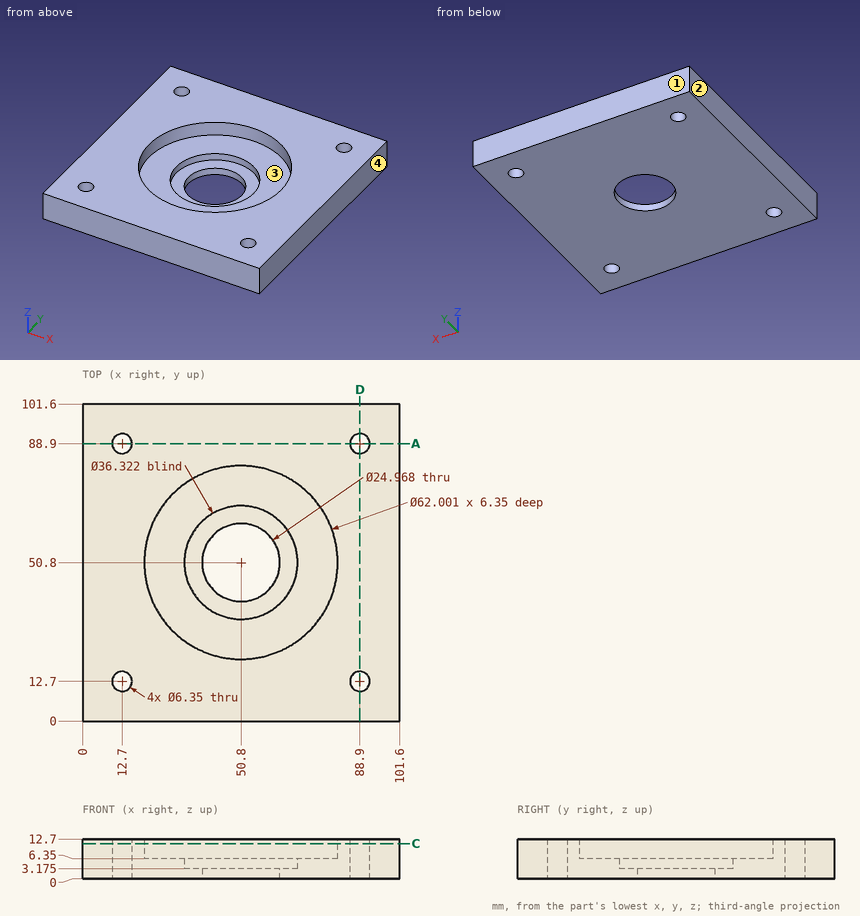
Here's the drawing with two shaded views (mm, measured from the low corner). I have some questions. Give positions to 0.01 mm unless a question says otherwise; leave off trailing zeros. Loops run counter-clockwise (first coordinate to the right, second up) from the corner with the lowest first, then second, coordinate; pieces in that order, holes last. Notation, with made-up numbers: (76.5, -11) - (90.5, -11) arc R16 cw to (90.5, 17) - close; hole circle Ø2 at (37.5, 29.5). An arc over 180 degrees is marked (long way). Answer in a Markdown table with one row per item. Add a question column.
Q1. Please list where these lines run through material, in increasing order: L1, parallel to Y at x = 88.9, z = 6.75 (1 decimal); L2, parallel to Y at x = 88, z = 10.5 (1 decimal). Write a range as from..to.
Q2. For pin 1 (8 mm diameter, centred on x = 26.5, y = 10.5, fed in from -Z); pin 2 (3 mm diameter, centred on x = 39.5, y = 50, fed in from +Z) (3 decimals), each with a flat end and sliding along its axis, tell me the tip position at first contact or that it passes through.
Q3. If we section it at C-C (z = 11.25): State how many separate pieces and enclosed holes the cut face has, plus the area to 3 significant figures.
Q4. We'd pull the mould along X, two halves only. Please class the marked faces 1, 2, 3 and 4: +X half, -X half, draft (parallel to the pull), parting line (faces both ways), or undercut.
Q5. If we section it at A-A (y = 88.9): List the corners of the cut face in (x, z) for me (1 decimal), plus the area to 3 significant figures.
The answers:
| question | item | result |
|---|---|---|
| 1 | L1 | y = 0..9.5, 15.9..85.7, 92.1..101.6 |
| 1 | L2 | y = 0..9.7, 15.7..85.9, 91.9..101.6 |
| 2 | pin 1 | stops at z = 0 |
| 2 | pin 2 | stops at z = 3.175 |
| 3 | separate pieces | 1 |
| 3 | enclosed holes | 5 |
| 3 | area | 7,180 mm^2 |
| 4 | face 1 | draft |
| 4 | face 2 | -X half |
| 4 | face 3 | undercut |
| 4 | face 4 | +X half |
| 5 | outline | (0, 0) - (9.5, 0) - (9.5, 12.7) - (0, 12.7) - close; (15.9, 0) - (85.7, 0) - (85.7, 12.7) - (15.9, 12.7) - close; (92.1, 0) - (101.6, 0) - (101.6, 12.7) - (92.1, 12.7) - close |
| 5 | area | 1,130 mm^2 |
